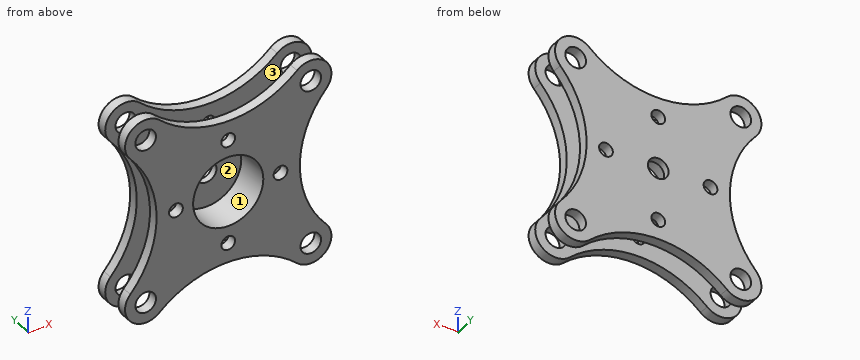
from build123d import *

# Parameters (mm, degrees)
SKETCH1_R           = 27.5
SKETCH1_R_2         = 7.5
SKETCH1_R_3         = 5
BOSS_EXTRUDE1_DEPTH = 7.5
SKETCH2_R           = 27.5
BOSS_EXTRUDE2_DEPTH = 30
SKETCH3_R           = 25.5
CUT_EXTRUDE1_DEPTH  = 25
SKETCH4_R           = 7.5
CUT_EXTRUDE2_DEPTH  = 25


with BuildPart() as part:
    # Sketch1 → Boss-Extrude1 (new body)
    with BuildSketch(Plane(origin=(0, 0, 0), x_dir=(1, 0, 0), z_dir=(0, 1, 0))):
        with BuildLine():
            ThreePointArc((-50, 71.180339887), (-70.606601718, 70.606601718), (-71.180339887, 50))
            ThreePointArc((-71.180339887, 50), (-52.082039325, 0), (-71.180339887, -50))
            ThreePointArc((-71.180339887, -50), (-70.606601718, -70.606601718), (-50, -71.180339887))
            ThreePointArc((-50, -71.180339887), (0, -52.082039325), (50, -71.180339887))
            ThreePointArc((50, -71.180339887), (70.606601718, -70.606601718), (71.180339887, -50))
            ThreePointArc((71.180339887, -50), (52.082039325, 0), (71.180339887, 50))
            ThreePointArc((71.180339887, 50), (70.606601718, 70.606601718), (50, 71.180339887))
            ThreePointArc((50, 71.180339887), (0, 52.082039325), (-50, 71.180339887))
        make_face()
        Circle(SKETCH1_R, mode=Mode.SUBTRACT)
        with Locations((-60, 60)):
            Circle(SKETCH1_R_2, mode=Mode.SUBTRACT)
        with Locations((60, 60)):
            Circle(SKETCH1_R_2, mode=Mode.SUBTRACT)
        with Locations((-60, -60)):
            Circle(SKETCH1_R_2, mode=Mode.SUBTRACT)
        with Locations((60, -60)):
            Circle(SKETCH1_R_2, mode=Mode.SUBTRACT)
        with Locations((0, 38)):
            Circle(SKETCH1_R_3, mode=Mode.SUBTRACT)
        with Locations((-38, 0)):
            Circle(SKETCH1_R_3, mode=Mode.SUBTRACT)
        with Locations((0, -38)):
            Circle(SKETCH1_R_3, mode=Mode.SUBTRACT)
        with Locations((38, 0)):
            Circle(SKETCH1_R_3, mode=Mode.SUBTRACT)
    boss_extrude1 = extrude(amount=-BOSS_EXTRUDE1_DEPTH)

    # Sketch2 → Boss-Extrude2 (add)
    with BuildSketch(Plane(origin=(0, 0, 0), x_dir=(1, 0, 0), z_dir=(0, 1, 0))):
        Circle(SKETCH2_R)
    extrude(amount=-BOSS_EXTRUDE2_DEPTH)

    # Sketch3 → Cut-Extrude1 (cut)
    with BuildSketch(Plane.XZ.offset(30)):
        Circle(SKETCH3_R)
    extrude(amount=-CUT_EXTRUDE1_DEPTH, mode=Mode.SUBTRACT)

    # Sketch4 → Cut-Extrude2 (cut)
    with BuildSketch(Plane.XZ.offset(5)):
        Circle(SKETCH4_R)
    extrude(amount=-CUT_EXTRUDE2_DEPTH, mode=Mode.SUBTRACT)

    # Mirror1: Boss-Extrude1 across plane
    add(boss_extrude1.mirror(Plane.ZX.offset(-15)))


solid = part.part
Can you work these out from the model? Positions are in its coordinate system, mm. Face numbers are marked on the shaded views. Give positions to 0.01 mm unless a question says otherwise; leave off trailing zeros. Loops run counter-clockwise (first coordinate to the right, second up) from the corner with the lowest first, then second, coordinate; pieces in that order, holes last. Notation, with made-up numbers: (54.5, -14.75) - (88.5, -14.75) arc R25 ccw to (88.5, 10.25) - close; hole circle Ø5 at (78.25, 40). An arc over 180 degrees is marked (long way). Answer as a JSON object with one key per item and string values.
Q1. Will these pins go through, and if not, where does the flat tip stop? P1, Ø3, axis at x = 41.5, y = -25.5, coming from the -Z side; P2, Ø1, axis at x = 56.5, y = -25.5, coming from the +Z side; P3, Ø1.5, axis at y = -24, z = -43.5, coming from the -X side.
Geometry says:
{"P1": "z = -65.63", "P2": "z = 74.7", "P3": "x = -66.53"}
Q2. If I drill on L1, parallel to Z at x = -58.5, y = -5.75; L2, parallel to Y at x = -11.5, z = -43; L3, parallel to Z at x = -59, y = -6.25, over which ranges is the centre line in solid material (lowest first)?
Geometry says:
{"L1": "-74.92 to -67.35, -52.65 to -30.36, 30.36 to 52.65, 67.35 to 74.92", "L2": "-30 to -22.5, -7.5 to 0", "L3": "-74.97 to -67.43, -52.57 to -31.46, 31.46 to 52.57, 67.43 to 74.97"}
Q3. Imagine slicing it at A-A on y = -24.5. Give the number of separate pieces and of enclosed holes in the cut face, plus the area to 3 significant figures.
Geometry says:
{"separate pieces": "1", "enclosed holes": "9", "area": "12,400 mm²"}
Q4. Imagine slicing it at D-D on z = 38. Write out the boundary of the cut face in (x, y).
Geometry says:
{"outline": "(-62.42, -30) - (-5, -30) - (-5, -22.5) - (-62.42, -22.5) - close; (-62.42, -7.5) - (-5, -7.5) - (-5, 0) - (-62.42, 0) - close; (5, -30) - (62.42, -30) - (62.42, -22.5) - (5, -22.5) - close; (5, -7.5) - (62.42, -7.5) - (62.42, 0) - (5, 0) - close"}
Q5. If we mould it in two halves opening along Z, with no side actions, what happens to the marked faces 1, 2 and 3? For each: pulls with the +Z half, pulls with the -Z half, needs draft (parallel to the pull), parting line crosses it, or undercut.
Geometry says:
{"face 1": "undercut", "face 2": "undercut", "face 3": "needs draft"}
